Here's how the part is built. I have some questions about the finished solid (model axes, mm). Round coordinates to 2 decimals unless told otherwise and drop trailing zeros. Write each loop counter-clockwise with the first axis right and the second up, starting at its lowest first coordinate (ties: lowest second). Pieces come first, ordered by that corner, then holes. Notation, with made-up numbers: (48, 69) -> (70, 69) arc R23 ccw to (70, 81) -> close; hole circle Ø6 at (55.5, 49.5). An arc over 180 degrees is marked (long way). Answer in a Markdown table with one row per item.
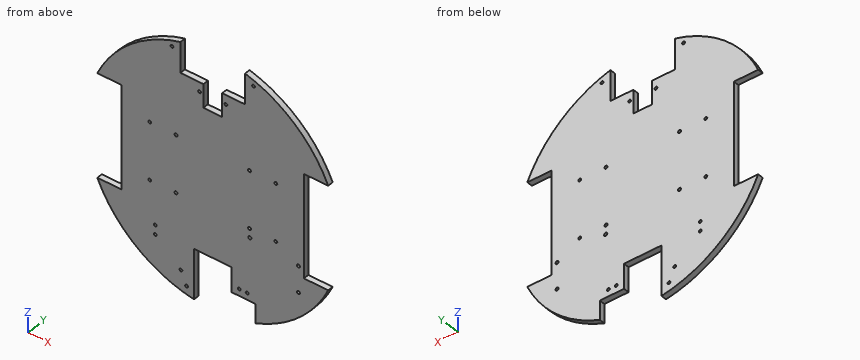
from build123d import *

# Parameters (mm, degrees)
ESQUISSE1_R                   = 135
BOSS_EXTRU_1_DEPTH            = 6
ESQUISSE2_W                   = 112.183682252
ESQUISSE2_H                   = 110
ESQUISSE2_W_2                 = 110.90382882
ENL_V_MAT_EXTRU_12_DEPTH      = 10
ENL_V_MAT_EXTRU_13_DEPTH      = 183.92348127
ENL_V_MAT_EXTRU_14_DEPTH      = 182.826840703
ENL_V_MAT_EXTRU_14_DEPTH_BACK = 182.826840703
ESQUISSE4_R                   = 1.653250653
ESQUISSE4_R_2                 = 1.624051272
ESQUISSE4_R_3                 = 1.712018077
ESQUISSE4_R_4                 = 1.6
ESQUISSE4_R_5                 = 1.599999728
ESQUISSE4_R_6                 = 1.599999892
ESQUISSE4_R_7                 = 1.599999865
ESQUISSE4_R_8                 = 1.599999855
ESQUISSE4_R_9                 = 1.5


with BuildPart() as part:
    # Esquisse1 → Boss.-Extru.1 (new body)
    with BuildSketch(Plane(origin=(0, 0, 0), x_dir=(1, 0, 0), z_dir=(0, 1, 0))):
        with Locations(Location((0, 0, 0), (0, 0, 270))):
            Circle(ESQUISSE1_R)
    extrude(amount=BOSS_EXTRU_1_DEPTH)

    # Esquisse2 → Enlèv. mat.-Extru.12 (cut)
    with BuildSketch(Plane(origin=(0, 6, 0), x_dir=(1, 0, 0), z_dir=(0, 1, 0))):
        with Locations((153.380121185, 0)):
            Rectangle(ESQUISSE2_W, ESQUISSE2_H)
        with Locations((-152.740194469, 0)):
            Rectangle(ESQUISSE2_W_2, ESQUISSE2_H)
    extrude(amount=-ENL_V_MAT_EXTRU_12_DEPTH, mode=Mode.SUBTRACT)

    # Esquisse3 → Enlèv. mat.-Extru.13 (cut, through all)
    with BuildSketch(Plane(origin=(0, 6, 0), x_dir=(1, 0, 0), z_dir=(0, 1, 0))):
        with BuildLine():
            Line((45.835319933, 106.66240667), (45.835319933, 126.980799519))
            ThreePointArc((45.835319933, 126.980799519), (23.265769543, 132.980088613), (0, 135))
            ThreePointArc((0, 135), (-10.027701736, 134.627059679), (-20, 133.510299228))
            Line((-20, 133.510299228), (-20, 80.28740667))
            Line((-20, 80.28740667), (20, 80.28740667))
            Line((20, 80.28740667), (20, 106.66240667))
            Line((20, 106.66240667), (45.835319933, 106.66240667))
        make_face()
        with BuildLine():
            Line((34.5, -98), (10, -98))
            Line((10, -98), (10, -73))
            Line((10, -73), (-10, -73))
            Line((-10, -73), (-10, -98))
            Line((-10, -98), (-34.5, -98))
            Line((-34.5, -98), (-34.5, -130.517240241))
            ThreePointArc((-34.5, -130.517240241), (-17.395007438, -133.874619388), (0, -135))
            ThreePointArc((0, -135), (17.395007438, -133.874619388), (34.5, -130.517240241))
            Line((34.5, -130.517240241), (34.5, -98))
        make_face()
    extrude(amount=-ENL_V_MAT_EXTRU_13_DEPTH, mode=Mode.SUBTRACT)

    # Esquisse4 → Enlèv. mat.-Extru.14 (cut, two sides: drawn at the far end of the back side and taken through both)
    with BuildSketch(Plane(origin=(0, 6, 0), x_dir=(1, 0, 0), z_dir=(0, 1, 0)).offset(-ENL_V_MAT_EXTRU_14_DEPTH_BACK)):
        with Locations(Location((91.525914299, 44.710203818, 0), (0, 0, 270))):
            Circle(ESQUISSE4_R)
        with Locations(Location((91.529697638, 72.638042273, 0), (0, 0, 270))):
            Circle(ESQUISSE4_R_2)
        with Locations(Location((39.606920151, 39.974167075, 0), (0, 0, 270))):
            Circle(ESQUISSE4_R_3)
        with Locations(Location((67.288280059, 30.548697725, 0), (0, 0, 270))):
            Circle(ESQUISSE4_R_4)
        with Locations(Location((39.288280059, 30.412294197, 0), (0, 0, 270))):
            Circle(ESQUISSE4_R_4)
        with Locations(Location((39.288280059, -30.547108673, 0), (0, 0, 270))):
            Circle(ESQUISSE4_R_5)
        with Locations(Location((67.288280059, -30.547108757, 0), (0, 0, 270))):
            Circle(ESQUISSE4_R_6)
        with Locations(Location((-39.288280059, -30.412294197, 0), (0, 0, 270))):
            Circle(ESQUISSE4_R_4)
        with Locations(Location((-67.288280059, -30.548697725, 0), (0, 0, 270))):
            Circle(ESQUISSE4_R_4)
        with Locations(Location((-67.288280059, 30.547108757, 0), (0, 0, 270))):
            Circle(ESQUISSE4_R_7)
        with Locations(Location((-39.288280059, 30.547108674, 0), (0, 0, 270))):
            Circle(ESQUISSE4_R_8)
        with Locations(Location((-61.462852102, 85.131040367, 0), (0, 0, 270))):
            Circle(ESQUISSE4_R_9)
        with Locations(Location((-61.462852102, 75.131040367, 0), (0, 0, 270))):
            Circle(ESQUISSE4_R_9)
        with Locations(Location((-28, 123.28740667, 0), (0, 0, 270))):
            Circle(ESQUISSE4_R_9)
        with Locations(Location((-34, 109.28740667, 0), (0, 0, 270))):
            Circle(ESQUISSE4_R_9)
        with Locations(Location((28.333333333, 99.41740667, 0), (0, 0, 270))):
            Circle(ESQUISSE4_R_9)
        with Locations(Location((36.666666667, 99.41740667, 0), (0, 0, 270))):
            Circle(ESQUISSE4_R_9)
        with Locations(Location((43.5, -121.562248636, 0), (0, 0, 270))):
            Circle(ESQUISSE4_R_9)
        with Locations(Location((-43.5, -121.562248636, 0), (0, 0, 270))):
            Circle(ESQUISSE4_R_9)
        with Locations(Location((14.08, -88, 0), (0, 0, 270))):
            Circle(ESQUISSE4_R_9)
        with Locations(Location((-14.07013432, -88, 0), (0, 0, 270))):
            Circle(ESQUISSE4_R_9)
    extrude(amount=ENL_V_MAT_EXTRU_14_DEPTH + ENL_V_MAT_EXTRU_14_DEPTH_BACK, mode=Mode.SUBTRACT)


solid = part.part
1) For pin 1 (2.5 mm diameter, centred on x = 39.29, z = 30.55, fed in from +Y); pin 2 (3 mm diameter, centred on y = 3.5, z = 117.5, fed in from +X); pin 3 (1.8 mm diameter, centred on y = 4, z = -117, fed in from -X); pin 4 (3 mm diameter, centred on y = 0.5, z = 79, fed in from +X), each with a flat end and sliding along its axis, tell me the tip position at first contact or that it passes through.
Response:
| item | result |
|---|---|
| pin 1 | passes through |
| pin 2 | stops at x = 69.06 |
| pin 3 | stops at x = -68.89 |
| pin 4 | stops at x = 110.54 |
2) I need wall thicknesses on line 1 (X direction, y = 0.55, z = -99); line 2 (Z direction, x = -40, y = 5.4); line 3 (X direction, y = 4.45, z = 6.5). Which ranges of each line are inside material? Lowest first, please. Write a range as [from, to].
Response:
| item | result |
|---|---|
| line 1 | x = [-91.78, -20], [20, 26.89], [29.77, 35.23], [38.11, 91.78] |
| line 2 | z = [-128.94, -31.98], [-29.11, 28.98], [31.85, 128.94] |
| line 3 | x = [-97.29, 97.29] |
3) I want a section at A-A, the plane z = -117. List the corners of the cut face in (x, y) for me, and give its area (3 significant figures).
Response:
| item | result |
|---|---|
| outline | (-67.35, 0) -> (-20, 0) -> (-20, 6) -> (-67.35, 6) -> close; (45.84, 0) -> (67.35, 0) -> (67.35, 6) -> (45.84, 6) -> close |
| area | 413 mm^2 |
4) I want a section at B-B, the plane z = 17. List the corners of the cut face in (x, y) for me.
Response:
| item | result |
|---|---|
| outline | (-97.29, 0) -> (97.29, 0) -> (97.29, 6) -> (-97.29, 6) -> close |
5) I want a section at D-D, the plane x = -52.5. List the corners of the cut face in (y, z) for me, and give its area (3 significant figures).
Response:
| item | result |
|---|---|
| outline | (0, -124.37) -> (6, -124.37) -> (6, 124.37) -> (0, 124.37) -> close |
| area | 1,490 mm^2 |
6) I want a section at C-C, the plane y = 2.4. Count the separate pieces of the cut face and the enclosed holes in it, and give its area (3 significant figures).
Response:
| item | result |
|---|---|
| separate pieces | 1 |
| enclosed holes | 21 |
| area | 43,900 mm^2 |
